Part model, mm, in its own coordinate system. Give positions to 0.01 mm unless a question says otherwise; leave off trailing zeros. Order: outer loops, then holes, each group sorted by start corner. A loop starts at its lowest first (then second) coordinate and runs counter-clockwise, first axis right, second up. Notation, with made-up numbers: M 13.5,72.25 L 33.5,72.25 A24 cw 33.5,110.25 Z; hole C 64,26 d3. An arc over 180 degrees is marked long. One line per question, with ' | ' between items.
```python
from build123d import *

# Parameters (mm, degrees)
F1_DEPTH = 1
F2_D     = 6


with BuildPart() as f1:
    # F0 (on Front) → F1 (new body)
    with BuildSketch(Plane.XZ):
        with BuildLine():
            Line((-54.0900086572, 22.3091947654), (-54.0900086572, -38.1908052346))
            ThreePointArc((-54.0900086572, -38.1908052346), (-52.0397561255, -43.1405527029), (-47.0900086572, -45.1908052346))
            Line((-47.0900086572, -45.1908052346), (-36.0900086572, -45.1908052346))
            ThreePointArc((-36.0900086572, -45.1908052346), (-31.1402611889, -43.1405527029), (-29.0900086572, -38.1908052346))
            Line((-29.0900086572, -38.1908052346), (-29.0900086572, -2.6908052346))
            ThreePointArc((-29.0900086572, -2.6908052346), (-27.0397561255, 2.2589422338), (-22.0900086572, 4.3091947654))
            Line((-22.0900086572, 4.3091947654), (13.4099913428, 4.3091947654))
            ThreePointArc((13.4099913428, 4.3091947654), (18.3597388111, 6.3594472971), (20.4099913428, 11.3091947654))
            Line((20.4099913428, 11.3091947654), (20.4099913428, 22.3091947654))
            ThreePointArc((20.4099913428, 22.3091947654), (18.3597388111, 27.2589422338), (13.4099913428, 29.3091947654))
            Line((13.4099913428, 29.3091947654), (-47.0900086572, 29.3091947654))
            ThreePointArc((-47.0900086572, 29.3091947654), (-52.0397561255, 27.2589422338), (-54.0900086572, 22.3091947654))
        make_face()
    extrude(amount=F1_DEPTH)

    # F2 (through all)
    with Locations(Plane(origin=(0, 0, 0), x_dir=(1, 0, 0), z_dir=(0, 1, 0))):
        with Locations((-41.5900086572, -16.8091947654), (8.4099913428, -16.8091947654), (-41.5900086572, 33.1908052346)):
            Hole(F2_D / 2)


solid = f1.part
```
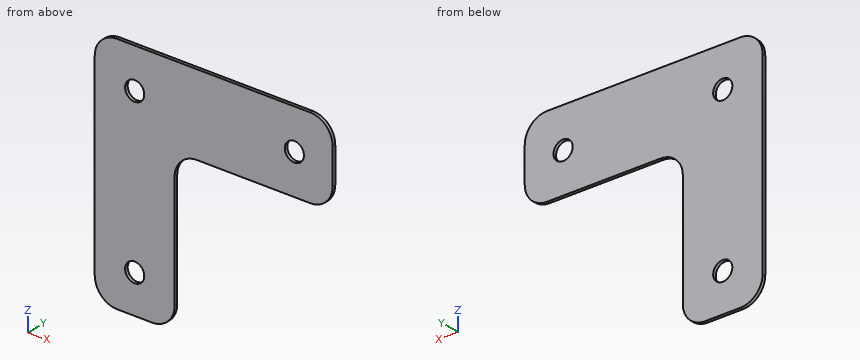
1. Slice it at D-D on x = -7.5. Give the cut face in (y, z), then the cut area to 3 significant figures.
Worked out:
outline: M -1,4.31 L 0,4.31 L 0,29.31 L -1,29.31 Z | area: 25.0 mm2
2. Slice it at A-A on x = 8.5. Give the cut face in (y, z).
Worked out:
outline: M -1,4.31 L 0,4.31 L 0,13.81 L -1,13.81 Z; M -1,19.81 L 0,19.81 L 0,29.31 L -1,29.31 Z
3. Slice it at C-C on y = -0.8. Give the cut face in (x, z), then the cut area to 3 significant figures.
Worked out:
outline: M -54.09,-38.19 A7 ccw -47.09,-45.19 L -36.09,-45.19 A7 ccw -29.09,-38.19 L -29.09,-2.69 A7 cw -22.09,4.31 L 13.41,4.31 A7 ccw 20.41,11.31 L 20.41,22.31 A7 ccw 13.41,29.31 L -47.09,29.31 A7 ccw -54.09,22.31 Z; hole C -41.59,-33.19 d6; hole C -41.59,16.81 d6; hole C 8.41,16.81 d6 | area: 2,970 mm2
4. Probe L1, parallel to X at y = -0.65, z = 16.5; L2, parallel to X at y = -0.85, z = -33.5; L3, parallel to Z at x = 2.5, y = -0.3. List the from-to ranges inside material, lowest first. Write a range as from..to.
Worked out:
L1: x = -54.09..-44.57, -38.61..5.43, 11.39..20.41 | L2: x = -54.09..-44.57, -38.61..-29.09 | L3: z = 4.31..29.31
5. Drop flat-ended pins along their axis: pin 1 (12 mm diameter, centred on x = -45, z = 0, fed in from +Y); pin 2 (0.5 mm diameter, centred on x = -7.5, y = -0.5, fed in from -Z). Give the stop position or say it passes through.
Worked out:
pin 1: stops at y = 0 | pin 2: stops at z = 4.31
6. Slice it at B-B on z = -35. Give the cut face in (x, y).
Worked out:
outline: M -54.09,-1 L -43.98,-1 L -43.98,0 L -54.09,0 Z; M -39.2,-1 L -29.09,-1 L -29.09,0 L -39.2,0 Z
